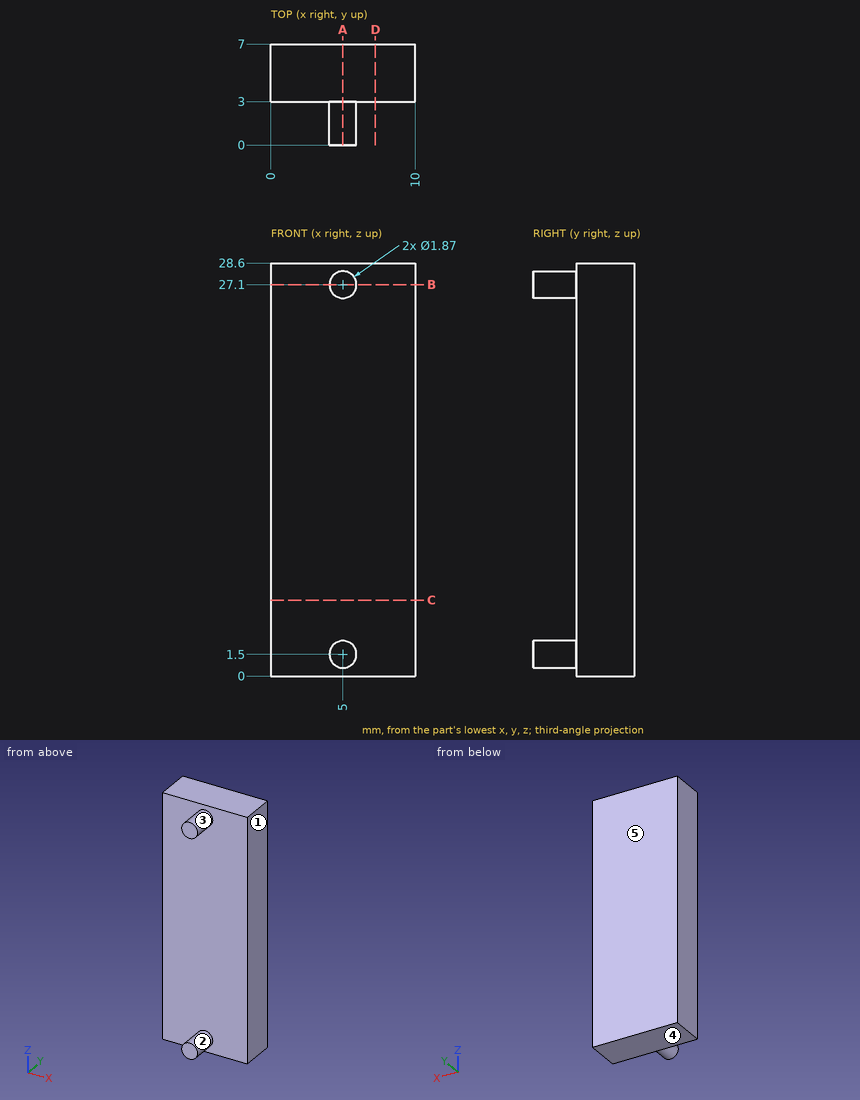
Here's the drawing with two shaded views (mm, measured from the low corner). I have some questions. A direction names the side the tool comes from. Coordinates: 2 decimals unless noted, no trailing zeros. Order: outer loops, then holes, each group sorted by start corner. A loop starts at its lowest first (then second) coordinate and runs counter-clockwise, first axis right, second up. Notation, with made-up numbers: (-30, 26.25) - (9, 26.25) arc R19 cw to (9, 42.25) - close; hole circle Ø11 at (32, 84). An arc over 180 degrees is marked (long way). Answer in a Markdown table with one row per item. Add a question column.
(1) If we section it at B-B, the plane z = 27.1: Please give me the cut outline in (x, y) (3 decimals), then the cut area to 3 significant figures.
(2) If we section it at A-A, the plane x = 5: Please give me the cut outline in (y, z) (3 decimals).
(3) Will these pins go through, and if not, where does the flat tip stop? pin 1 (1.5 mm diameter, centred on x = 5, z = 17.5, fed in from -Y); pin 2 (4 mm diameter, centred on x = 6.5, y = 2.5, fed in from -Z).
(4) I need wall thicknesses on L1, parallel to Y at x = 1.5, z = 5. Which ranges of the line are inside material? Lowest first, please.
(5) If we section it at D-D, the plane x = 7.25: Please give me the cut outline in (y, z).
(6) On a 3-axis mill with a long thin cutter (end or side, diameter ignored), from which of +Z, -Z, +X, -X, +Y, -Y can I reach the whole of each face in a straight line? I mean the marked faces 1 and 2. Say none if no direction works.
(7) If we section it at C-C, the plane z = 5.25: Please give me the cut outline in (x, y), then the cut area to 3 significant figures.
(8) If we mould it in two halves opening along Z, with no side actions, what happens to the marked faces 3, 4 and 5? For each: released by +Z, released by -Z, zero draft, split by the parting line, or undercut.
Results are:
| question | item | result |
|---|---|---|
| 1 | outline | (0, 3) - (4.065, 3) - (4.065, 0) - (5.935, 0) - (5.935, 3) - (10, 3) - (10, 7) - (0, 7) - close |
| 1 | area | 45.6 mm2 |
| 2 | outline | (0, 0.565) - (3, 0.565) - (3, 0) - (7, 0) - (7, 28.6) - (3, 28.6) - (3, 28.035) - (0, 28.035) - (0, 26.165) - (3, 26.165) - (3, 2.435) - (0, 2.435) - close |
| 3 | pin 1 | stops at y = 3 |
| 3 | pin 2 | stops at z = 0 |
| 4 | L1 | y = 3 to 7 |
| 5 | outline | (3, 0) - (7, 0) - (7, 28.6) - (3, 28.6) - close |
| 6 | face 1 | +Z, -Z, +X, +Y, -Y |
| 6 | face 2 | -Y |
| 7 | outline | (0, 3) - (10, 3) - (10, 7) - (0, 7) - close |
| 7 | area | 40.0 mm2 |
| 8 | face 3 | undercut |
| 8 | face 4 | released by -Z |
| 8 | face 5 | zero draft |
